Verification items for the finished model (mm, model axes). A direction names the side the tool comes from. Give positions to 0.01 mm unless a question says otherwise; leave off trailing zeros. Order: outer loops, then holes, each group sorted by start corner. A loop starts at its lowest first (then second) coordinate and runs counter-clockwise, first axis right, second up.
(1) Scan lines: L1, parallel to Y at x = -5, z = 9.5; L2, parallel to Z at x = 20, y = -30.5; L3, parallel to Z at x = -7.5, y = -8.5. Record each from-to range of solid material in increasing order.
(2) Sectioned sample at C-C on y = -13. Record the cut outline in (x, z).
(3) Sectioned sample at D-D on z = 14. Record the cut outline in (x, y), plus the area to 3 significant figures.
(4) Sectioned sample at A-A on z = 10.5. Record the cut outline in (x, y).
(5) Access from +Z, -Z, +X, -X, +Y, -Y to the whole of each face (thin tool, end or side, straight path). Record for faces 5 (the face through (-8.34, -44.43, 7.54)), 6 (the face through (11.42, -22.54, 7.51)).
(6) Mould release check, pull along Z, two halves, no side actions. Record for faces 1 (the face through (-10.81, -22.54, 7.73)), 2 (the face through (0, -43.18, 6)), 3 (the face through (0, 0, 6)), 4 (the face through (0, -23, 0)): pulls with the +Z half, pulls with the -Z half, needs draft (parallel to the pull), parting line crosses it, or undercut.
(7) Gauge pin test, flat ends, axial feed: pin 1 (8 mm diameter, centred on x = 2, z = 3, fed in from -Y); pin 2 (2 mm diameter, centred on x = -15, y = -13.5, fed in from +Z); pin 3 (2 mm diameter, centred on x = 5.5, y = -44.5, fed in from +Z); pin 4 (3.5 mm diameter, centred on x = 6.5, z = 5.5, fed in from -Y). Record the tip position at first contact, or that the pin passes through.
(8) Sectioned sample at B-B on x = 4. Record the cut outline in (y, z), plus the area to 3 significant figures.
```python
from build123d import *

# Parameters (mm, degrees)
F1_DEPTH = 45.72
F2_DEPTH = 43.18


with BuildPart() as f1:
    # F0 (on Front) → F1 (new body)
    with BuildSketch(Plane.XZ):
        Polygon((0, 15.24), (-21.933843, 0), (0, 0), (0, 1.903249), (-16.452903, 1.903249), (0, 13.335), align=None)
        Polygon((0, 1.903249), (0, 0), (22.516157, 0), (0, 15.24), (0, 13.335), (16.889705, 1.903249), align=None)
    extrude(amount=F1_DEPTH)

    # F0 (on Front) → F2 (join)
    with BuildSketch(Plane.XZ):
        Polygon((-16.452903, 1.903249), (0, 1.903249), (16.889705, 1.903249), (0, 13.335), align=None)
    extrude(amount=F2_DEPTH)


solid = f1.part
```
Ans:
1. L1: y = -43.18 to 0
1. L2: z = 0 to 1.7
1. L3: z = 0 to 10.03
2. outline: (-21.93, 0) - (22.52, 0) - (0, 15.24) - close
3. outline: (-1.78, -45.72) - (1.83, -45.72) - (1.83, 0) - (-1.78, 0) - close
3. area: 165 mm2
4. outline: (-6.82, -45.72) - (-4.08, -45.72) - (-4.08, -43.18) - (4.19, -43.18) - (4.19, -45.72) - (7, -45.72) - (7, 0) - (-6.82, 0) - close
5. face 5: -Y
5. face 6: +Z, +X, +Y, -Y
6. face 1: pulls with the +Z half
6. face 2: undercut
6. face 3: needs draft
6. face 4: pulls with the -Z half
7. pin 1: stops at y = -45.72
7. pin 2: stops at z = 5.51
7. pin 3: stops at z = 12.19
7. pin 4: stops at y = -43.18
8. outline: (-45.72, 0) - (0, 0) - (0, 12.53) - (-45.72, 12.53) - (-45.72, 10.63) - (-43.18, 10.63) - (-43.18, 1.9) - (-45.72, 1.9) - close
8. area: 551 mm2
